Geometry check sheet. Reference: drawing and pictorial views, mm from the part's lowest x, y, z. Give positions to 0.01 mm unless a question says otherwise; leave off trailing zeros. Write each loop counter-clockwise with the first axis right and the second up, starting at its lowest first coordinate (ties: lowest second). Pieces come first, ordered by that corner, then holes. Notation, with made-up numbers: (52, 12) -> (81, 12) arc R24 ccw to (81, 26) -> close; hole circle Ø2 at (-28.5, -21.5). An arc over 180 degrees is marked (long way). Answer as CSV lines item,"result".
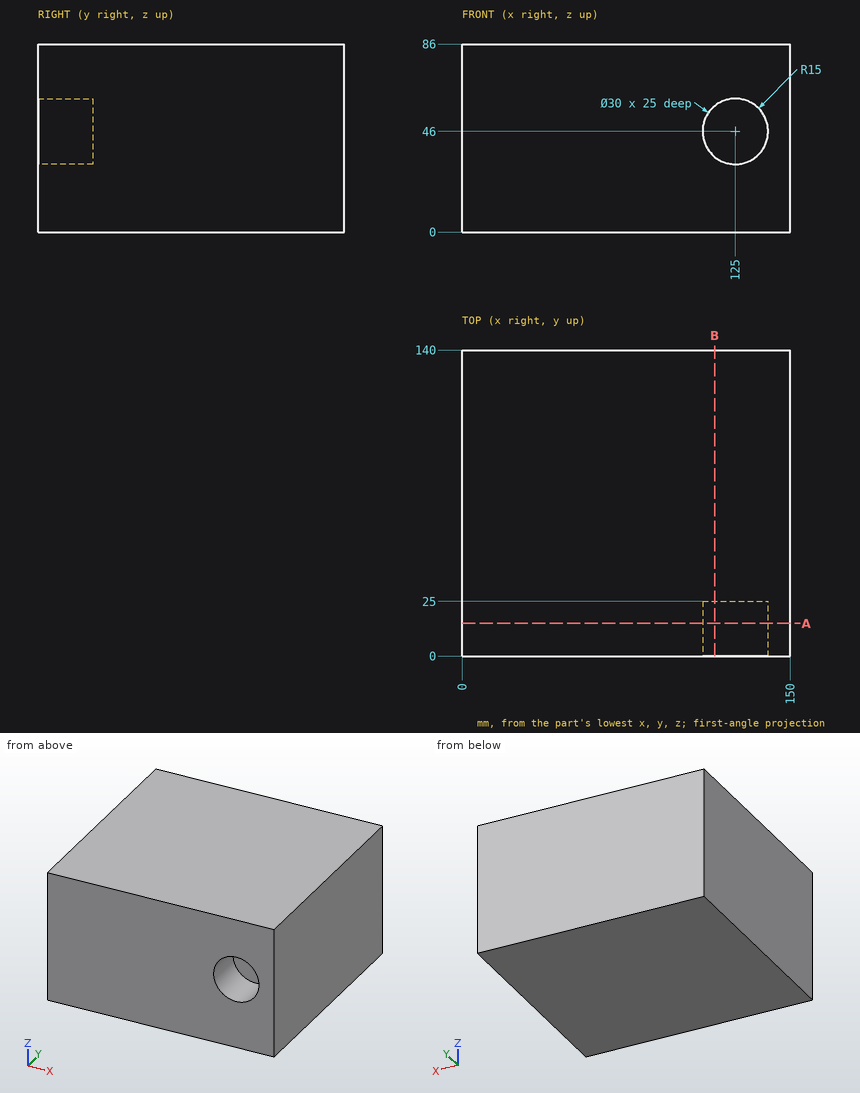
1) Section check A-A (y = 15). Record the boundary of the cut face in (x, z), and give its area (3 significant figures).
Reported:
outline,"(0, 0) -> (150, 0) -> (150, 86) -> (0, 86) -> close; hole (125, 61) arc R15 ccw (long way) to (140, 46) arc R15 ccw to start"
area,"12,200 mm²"
2) Section check B-B (x = 115.5). Record the boundary of the cut face in (y, z), and give its area (3 significant figures).
Reported:
outline,"(0, 0) -> (140, 0) -> (140, 86) -> (0, 86) -> (0, 57.61) -> (25, 57.61) -> (25, 34.39) -> (0, 34.39) -> close"
area,"11,500 mm²"
3) Scan lines: line 1 along Z through (x, y) = (125, 17); line 2 along X through (y, z) = (13, 46); line 3 along Y through (x, z) = (125, 39). Record each from-to range of solid material in increasing order.
Reported:
line 1,"0 to 31, 61 to 86"
line 2,"0 to 110, 140 to 150"
line 3,"25 to 140"
4) Depth check by flat-ended pin: pin 1 (18 mm diameter, centred on x = 125, z = 46, fed in from -Y). Enter the tip coordinate at first touch or a pass-through.
Reported:
pin 1,"y = 25"
